Check sheet for the modelled part. Datum: model origin and axes. Units: mm. A direction names the side the tool comes from. Round coordinates to 2 decimals unless told otherwise and drop trailing zeros. Order: outer loops, then holes, each group sorted by start corner. A loop starts at its lowest first (then second) coordinate and runs counter-clockwise, first axis right, second up.
Q1. Set-up check for faces 4 (the flat face through (13, -64.031, -11)), 5 (the flat face through (13, 28.924, -6)): record each of +Z, -Z, +X, -X, +Y, -Y from which the full face is reachable in a straight line by a thin tool's end or side.
Q2. Cross-section at D-D on z = 11. Record the cut outline in (x, y), then the cut area to 3 significant figures.
Q3. Cross-section at C-C on y = -57. Record the cut outline in (x, z).
Q4. Cross-section at A-A on z = -31.5. Record the cut outline in (x, y).
Q5. Depth check by flat-ended pin: P1, Ø1, axis at x = 14.5, y = 24.5, coming from the +Z side; P2, Ø1, axis at y = -52.5, z = -0.5, coming from the -X side; P3, Ø1.5, axis at x = 13.5, z = -64, coming from the +Y side. Enter the tip coordinate at first touch or a pass-through.
Q6. Mould release check, pull along X, two halves, no side actions. Record for faces 1 (the flat face through (13, -48.791, -7)), 2 (the cylindrical face through (15.75, -56.52, 21.25)), 3 (the cylindrical face through (0.765, -2.24, -67.883)): +X half, -X half, draft (parallel to the pull), parting line (faces both ways), or undercut.
Q7. Cross-section at B-B on x = 17.75. Record the cut outline in (y, z).
Q8. Scan lines: probe 1 along Y at (x, z) = (10.25, -19); probe 2 along Z at (x, y) = (16.75, -18.5); probe 3 along Z at (x, y) = (0.25, -20). Record each from-to range of solid material in increasing order.
from build123d import *

# Parameters (mm, degrees)
F0_W     = 77.7157761486
F0_H     = 10.8950532058
F1_DEPTH = 25.4
F2_R     = 7.62
F3_DEPTH = 127
F4_R     = 12.6365
F5_DEPTH = 25.4


with BuildPart() as f1:
    # F0 (on Right) → F1 (new body)
    with BuildSketch(Plane.YZ):
        Polygon((-48.7912997933, 31.7609666863), (-64.0312997933, 31.7609666863), (-64.0312997933, -55.3610383549), (-48.7912997933, -55.3610383549), (-48.7912997933, -44.4659851491), align=None)
        Polygon((28.9244763553, 31.7609666863), (28.9244763553, -44.4659851491), (28.9244763553, -55.3610383549), (44.1727048095, -55.3610383549), (44.1727048095, 31.7609666863), align=None)
        with Locations((-9.933411719, -49.913511752)):
            Rectangle(F0_W, F0_H)
    extrude(amount=F1_DEPTH)

    # F2 (on face) → F3 (cut)
    with BuildSketch(Plane.XZ.offset(64.0312997933)):
        with Locations((11.656133458, 14.8219969124)):
            Circle(F2_R)
    extrude(amount=-F3_DEPTH, mode=Mode.SUBTRACT)

    # F4 (on face) → F5 (join)
    with BuildSketch(Plane(origin=(0, 0, -55.3610383549), x_dir=(1, 0, 0), z_dir=(0, 0, -1))):
        with Locations((10.7927164063, 9.9292974919)):
            Circle(F4_R)
    extrude(amount=F5_DEPTH)


solid = f1.part
Results found:
1. face 4: +Z, -Z, +X, -X, -Y
1. face 5: +Z, +X, -X
2. outline: (0, -64.03) - (5.06, -64.03) - (5.06, -48.79) - (0, -48.79) - close; (0, 28.92) - (5.06, 28.92) - (5.06, 44.17) - (0, 44.17) - close; (18.25, -64.03) - (25.4, -64.03) - (25.4, -48.79) - (18.25, -48.79) - close; (18.25, 28.92) - (25.4, 28.92) - (25.4, 44.17) - (18.25, 44.17) - close
2. area: 372 mm2
3. outline: (0, -55.36) - (25.4, -55.36) - (25.4, 31.76) - (0, 31.76) - close; hole circle Ø15.24 at (11.66, 14.82)
4. outline: (0, -64.03) - (25.4, -64.03) - (25.4, -48.79) - (0, -48.79) - close; (0, 28.92) - (25.4, 28.92) - (25.4, 44.17) - (0, 44.17) - close
5. P1: stops at z = -44.47
5. P2: stops at x = 0
5. P3: stops at y = 2.55
6. face 1: draft
6. face 2: undercut
6. face 3: parting line
7. outline: (-64.03, -55.36) - (-20.48, -55.36) - (-20.48, -80.76) - (0.62, -80.76) - (0.62, -55.36) - (44.17, -55.36) - (44.17, 10.25) - (28.92, 10.25) - (28.92, -44.47) - (-48.79, -44.47) - (-48.79, 10.25) - (-64.03, 10.25) - close; (-64.03, 19.4) - (-48.79, 19.4) - (-48.79, 31.76) - (-64.03, 31.76) - close; (28.92, 19.4) - (44.17, 19.4) - (44.17, 31.76) - (28.92, 31.76) - close
8. probe 1: y = -64.03 to -48.79, 28.92 to 44.17
8. probe 2: z = -80.76 to -44.47
8. probe 3: z = -55.36 to -44.47
